Read the model definition and answer for the solid it produces. Units are mm, in the model's axes. Face numbers are marked on the shaded views. A direction names the side the tool comes from. Give positions to 0.01 mm unless a question says otherwise; leave off trailing zeros. Order: outer loops, then holes, each group sorted by start corner. A loop starts at its lowest first (then second) coordinate and runs counter-clockwise, first axis right, second up.
```python
from build123d import *

# Parameters (mm, degrees)
SKETCH1_W           = 150
SKETCH1_H           = 150
BOSS_EXTRUDE1_DEPTH = 50
SKETCH2_W           = 100
SKETCH2_H           = 100
BOSS_EXTRUDE2_DEPTH = 2000
SKETCH3_R           = 25
CUT_EXTRUDE1_DEPTH  = 25


with BuildPart() as part:
    # Sketch1 → Boss-Extrude1 (new body)
    with BuildSketch(Plane(origin=(0, 0, 0), x_dir=(1, 0, 0), z_dir=(0, 1, 0))):
        Rectangle(SKETCH1_W, SKETCH1_H)
    extrude(amount=BOSS_EXTRUDE1_DEPTH)

    # Sketch2 → Boss-Extrude2 (add)
    with BuildSketch(Plane.XZ):
        Rectangle(SKETCH2_W, SKETCH2_H)
    extrude(amount=BOSS_EXTRUDE2_DEPTH)

    # Sketch3 → Cut-Extrude1 (cut)
    with BuildSketch(Plane.XZ.offset(2000)):
        with Locations(Location((0, 0, 0), (0, 0, 270))):
            Circle(SKETCH3_R)
    extrude(amount=-CUT_EXTRUDE1_DEPTH, mode=Mode.SUBTRACT)


solid = part.part
```
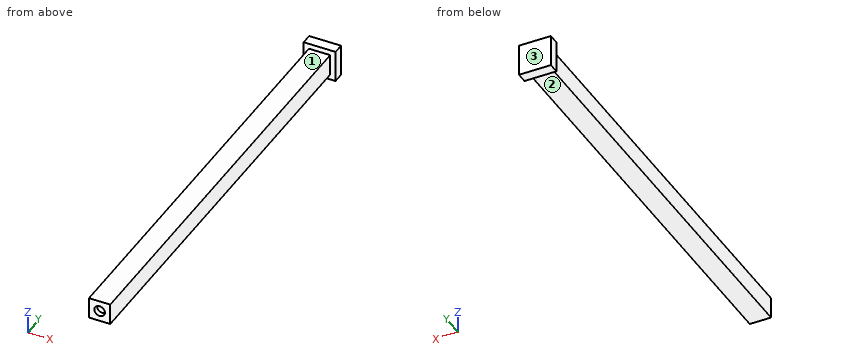
1) Consider L1, parallel to X at y = -1983, z = 0; L2, parallel to X at y = -265, z = 28. Determine where each line is inside the solid, lowest interval first.
Final values:
L1: x = -50 to -25, 25 to 50
L2: x = -50 to 50
2) The part is cut by section B-B on x = 0. Determine the outline of the cut face in (y, z).
Final values:
outline: (-2000, -50) - (0, -50) - (0, -75) - (50, -75) - (50, 75) - (0, 75) - (0, 50) - (-2000, 50) - (-2000, 25) - (-1975, 25) - (-1975, -25) - (-2000, -25) - close
3) A tool of negligible diameter and unlimited length cuts with its end or side. For the marked faces 1, 2 and 3, from which of +Z, -Z, +X, -X, +Y, -Y can it reach the whole face along a straight path? Write none if from no direction.
Final values:
face 1: +Z, +X, -X, -Y
face 2: -Z, +X, -X, -Y
face 3: +Z, -Z, +X, -X, +Y
4) The part is cut by section A-A on z = 0. Determine the outline of the cut face in (x, y), and give its area (3 significant figures).
Final values:
outline: (-75, 0) - (-50, 0) - (-50, -2000) - (-25, -2000) - (-25, -1975) - (25, -1975) - (25, -2000) - (50, -2000) - (50, 0) - (75, 0) - (75, 50) - (-75, 50) - close
area: 206,000 mm2
5) The part is cut by section C-C on y = -1268.5. Determine the outline of the cut face in (x, z), and give its area (3 significant figures).
Final values:
outline: (-50, -50) - (50, -50) - (50, 50) - (-50, 50) - close
area: 10,000 mm2
6) Given pin 1 (6 mm diameter, centred on y = -731.5, z = 8.5, fed in from +X); pin 2 (8 mm diameter, centred on x = 43.5, y = -370.5, fed in from -Z); pin 3 (2 mm diameter, centred on y = -1575.5, z = -11.5, fed in from -X), each flat-ended and moving along its own axis, determine where each tip first touches the part or whether it passes through.
Final values:
pin 1: stops at x = 50
pin 2: stops at z = -50
pin 3: stops at x = -50
